Could you check a few things on this model? Use its own coordinates, in mm. Face numbers are marked on the shaded views. A direction names the side the tool comes from. Round coordinates to 2 decimals unless told otherwise and drop trailing zeros. Write each loop counter-clockwise with the first axis right and the second up, starting at its lowest first coordinate (ties: lowest second). Pieces come first, ordered by that corner, then holes. Notation, with made-up numbers: M 59.5,71 L 112.5,71 A17 cw 112.5,94 Z; hole C 42,12 d1. An arc over 180 degrees is marked long. One line per item, written item: value. Start each with the question number.
(1) I want a section at D-D on y = -66.5. Please give me the cut outline in (x, z).
(2) I want a section at A-A on z = 23. Please give me the cut outline in (x, y).
(3) I want a section at B-B on y = 32. Please give me the cut outline in (x, z).
(4) Which directions (+Z, -Z, +X, -X, +Y, -Y) give clear straight access to the entire face, cutting with the end or side of a thin tool? Please do the marked faces 1 and 2.
(5) I want a section at C-C on x = -51. Please give me the cut outline in (y, z), and give its area (3 significant figures).
(6) If I drill on L1, parallel to Y at x = 0, z = 2.4; L2, parallel to Y at x = 57, z = 4.5; L3, parallel to Y at x = 9.5, z = 23, over which ranges is the centre line in solid material (lowest first)?
(7) I'm going to push flat-ended pins straight in: pin 1 Ø12 at (x, y) = (30, 69) entering from +Z; pin 2 Ø1.5 at (x, z) = (54.5, 3.5) entering from +Y; pin 3 Ø12 at (y, z) = (12, 10) entering from +X. Where does each tip first touch, or does it pass through?
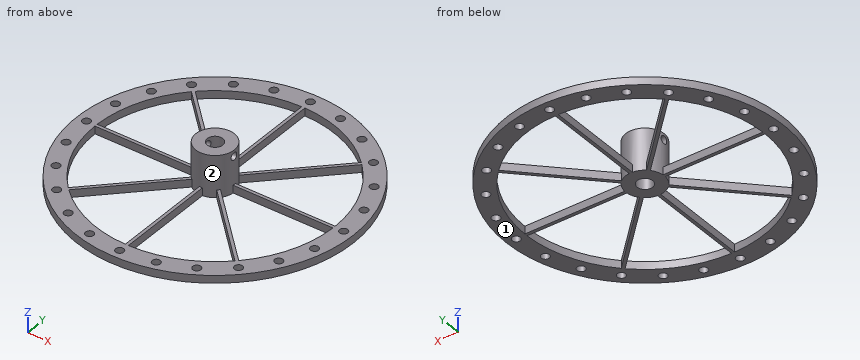
Autodesk Fusion 360 part; units mm, degrees
sketch "Sketch1" plane through (0, 0, 0) normal (0, 0, 1) x (1, 0, 0)
  line L0 (-1, 0) -> (-1, -77.5)
  line L1 (-0.4142, -1) -> (77.5, -1)
  line L2 (-1, 0) -> (-1, 77.5)
  line L3 (-0.4142, 1) -> (-55.5079, -54.0937)
  line L4 (0, 0) -> (77.5, 0) construction
  line L5 (0, 0) -> (0, 77.5) construction
  line L6 (0, 0) -> (-54.8008, -54.8008) construction
  line L7 (-2.4142, 1) -> (54.0937, -55.5079)
  line L8 (0, 0) -> (0, -77.5) construction
  line L9 (-0.4142, -1) -> (-55.5079, 54.0937)
  line L10 (0, -1) -> (-77.5, -1)
  line L11 (2.4142, 1) -> (55.5079, 54.0937)
  line L12 (0, 0) -> (77.5, 0) construction
  line L13 (0.7071, 0.7071) -> (-54.0937, 55.5079)
  line L14 (0, 0) -> (-54.8008, 54.8008) construction
  line L15 (2.4142, 1) -> (77.5, 1)
  line L16 (0, 1) -> (-77.5, 1)
  circle A0 centre (0, 0) radius 12.5
  line L17 (-2.4142, 1) -> (77.5, 1)
  line L18 (-0.4142, 1) -> (77.5, 1)
  line L19 (2.4142, -1) -> (77.5, -1)
  line L20 (-2.4142, -1) -> (77.5, -1)
  line L21 (0, 0) -> (-77.5, 0) construction
  circle A1 centre (0, 0) radius 5.05
  line L22 (1, 0) -> (1, -77.5)
  line L23 (0.4142, -1) -> (-54.0937, -55.5079)
  line L24 (0, 0) -> (54.8008, 54.8008) construction
  line L25 (1, 0) -> (1, 77.5)
  line L26 (0, 0) -> (77.5, 0) construction
  circle A2 centre (0, 0) radius 77.5
  line L27 (0, 0) -> (77.5, 0) construction
  circle A3 centre (0, 0) radius 90
  line L28 (0.4142, -1) -> (77.5, -1)
  line L29 (0, 0) -> (54.8008, -54.8008) construction
  line L30 (-2.4142, -1) -> (54.0937, 55.5079)
  line L31 (0, 0) -> (77.5, 0) construction
  line L32 (2.4142, -1) -> (55.5079, -54.0937)
  dimension "d42" = 1
  dimension "d43" = -1
  dimension "d44" = 1
  dimension "d45" = -1
  dimension "d46" = 1
  dimension "d47" = -1
  dimension "d48" = 1
  dimension "d49" = -1
  dimension "d50" = 1
  dimension "d51" = -1
  dimension "d52" = 1
  dimension "d53" = -1
  dimension "d54" = 1
  dimension "d55" = -1
  dimension "d33" = 10.1
  dimension "d35" = 180
  dimension "d37" = 155
  dimension "d38" = 45
  dimension "d39" = 45
  dimension "d40" = 135
  dimension "d41" = 135
  dimension "d56" = 25
extrude "Extrude1" add sketch "Sketch1" along normal blind 27 contours L0 A0 A1 L22 | L0 A0 A1 L23 | L3 A0 A1 L23 | L3 L10 A0 A1 | L10 L16 A0 A1 | L9 L16 A0 A1 | L9 L13 A0 A1 | L2 L13 A0 A1 | L2 A0 A1 L25 | L7 A0 A1 L22 | L7 A0 A1 L32 | A0 A1 L25 L30 | L11 A0 A1 L30 | L1 A0 L19 L20 A1 L28 L32 | L11 L15 A0 L17 L18 A1 | L1 L15 A0 L17 L18 L19 L20 A1 L28
extrude "Extrude2" add sketch "Sketch1" along normal blind 5 contours L0 A0 L22 A2 | L3 A0 L23 A2 | L10 L16 A0 A2 | L9 L13 A0 A2 | L2 A0 L25 A2 | L7 A0 A2 L32 | L11 A0 A2 L30 | L1 L15 A0 L17 L18 L19 L20 A2 L28 | A3
sketch "Sketch2" plane through (0, 0, 5) normal (0, 0, 1) x (-1, 0, 0)
  arc A0 (1, 12.4599) -> (-1, 12.4599) centre (0, 0) ccw
  line L0 (1, 12.4599) -> (1, 77.4935)
  arc A1 (54.0891, 55.5033) -> (1, 77.4935) centre (0, 0) ccw
  line L1 (54.0891, 55.5033) -> (8.1034, 9.5176)
  arc A2 (9.5176, 8.1034) -> (8.1034, 9.5176) centre (0, 0) ccw
  line L2 (9.5176, 8.1034) -> (55.5033, 54.0891)
  arc A3 (77.4935, 1) -> (55.5033, 54.0891) centre (0, 0) ccw
  line L3 (77.4935, 1) -> (12.4599, 1)
  arc A4 (12.4599, -1) -> (12.4599, 1) centre (0, 0) ccw
  line L4 (12.4599, -1) -> (77.4935, -1)
  arc A5 (55.5033, -54.0891) -> (77.4935, -1) centre (0, 0) ccw
  line L5 (55.5033, -54.0891) -> (9.5176, -8.1034)
  arc A6 (8.1034, -9.5176) -> (9.5176, -8.1034) centre (0, 0) ccw
  line L6 (8.1034, -9.5176) -> (54.0891, -55.5033)
  arc A7 (1, -77.4935) -> (54.0891, -55.5033) centre (0, 0) ccw
  line L7 (1, -77.4935) -> (1, -12.4599)
  arc A8 (-1, -12.4599) -> (1, -12.4599) centre (0, 0) ccw
  line L8 (-1, -12.4599) -> (-1, -77.4935)
  arc A9 (-54.0891, -55.5033) -> (-1, -77.4935) centre (0, 0) ccw
  line L9 (-54.0891, -55.5033) -> (-8.1034, -9.5176)
  arc A10 (-9.5176, -8.1034) -> (-8.1034, -9.5176) centre (0, 0) ccw
  line L10 (-9.5176, -8.1034) -> (-55.5033, -54.0891)
  arc A11 (-77.4935, -1) -> (-55.5033, -54.0891) centre (0, 0) ccw
  line L11 (-77.4935, -1) -> (-12.4599, -1)
  arc A12 (-12.4599, 1) -> (-12.4599, -1) centre (0, 0) ccw
  line L12 (-12.4599, 1) -> (-77.4935, 1)
  arc A13 (-55.5033, 54.0891) -> (-77.4935, 1) centre (0, 0) ccw
  line L13 (-55.5033, 54.0891) -> (-9.5176, 8.1034)
  arc A14 (-8.1034, 9.5176) -> (-9.5176, 8.1034) centre (0, 0) ccw
  line L14 (-8.1034, 9.5176) -> (-54.0891, 55.5033)
  arc A15 (-1, 77.4935) -> (-54.0891, 55.5033) centre (0, 0) ccw
  line L15 (-1, 77.4935) -> (-1, 12.4599)
  circle A16 centre (0, 0) radius 90
  line L16 (-77.5, 0) -> (-83.75, 0) construction
  circle A17 centre (-83.75, 0) radius 2.65
  point P0 (-77.5, 0)
  dimension "d28" = 6.25
  dimension "d29" = 5.3
hole "Hole1" at (83.75, 0, 5) direction (0, 0, -1) diameter 5.3 depth 10 tip angle 180
pattern_circular "C-Pattern1" count 24 over 360 about axis through (0, 0, 0) along (0, 0, 1) of "Hole1"
ref_plane "WorkPlane1" through (12.5, 0, 19.1773) normal (1, 0, 0) x (0, -1, 0)
ref_plane "WorkPlane2" through (-12.5, 0, 14.5915) normal (-1, 0, 0) x (0, 1, 0)
ref_plane "WorkPlane3" through (0, 0, 14.5915) normal (-1, 0, 0) x (0, 1, 0)
sketch "Sketch3" plane through (0, 0, 14.5915) normal (-1, 0, 0) x (0, 1, 0)
  line L0 (-12.5, -12.4085) -> (12.5, -12.4085)
  line L1 (0, -12.4085) -> (0, -8.4085)
  circle A0 centre (0, -8.4085) radius 2.5
  dimension "d59" = 4
  dimension "d60" = 5
extrude "Extrude3" cut sketch "Sketch3" along normal blind 16 and the other way blind 18
equation "d28 = ( 12.500 / 2 ) * 1 mm"
Found:
1. outline: M -60.64,0 L -39.8,0 L -39.8,5 L -60.64,5 Z; M -1,0 L 1,0 L 1,5 L -1,5 Z; M 39.8,0 L 60.64,0 L 60.64,5 L 39.8,5 Z
2. outline: M -12.25,-2.5 A12.5 ccw 12.25,-2.5 L 4.39,-2.5 A5.05 cw -4.39,-2.5 Z; M -12.25,2.5 L -4.39,2.5 A5.05 cw 4.39,2.5 L 12.25,2.5 A12.5 ccw Z
3. outline: M -84.12,0 L -70.59,0 L -70.59,5 L -84.12,5 Z; M -33.41,0 L -30.59,0 L -30.59,5 L -33.41,5 Z; M -1,0 L 1,0 L 1,5 L -1,5 Z; M 30.59,0 L 33.41,0 L 33.41,5 L 30.59,5 Z; M 70.59,0 L 84.12,0 L 84.12,5 L 70.59,5 Z
4. face 1: -Z, +X, -X, +Y, -Y
4. face 2: +Z
5. outline: M -74.16,0 L -58.35,0 L -58.35,5 L -74.16,5 Z; M -52.41,0 L -49.59,0 L -49.59,5 L -52.41,5 Z; M -1,0 L 1,0 L 1,5 L -1,5 Z; M 49.59,0 L 52.41,0 L 52.41,5 L 49.59,5 Z; M 58.35,0 L 74.16,0 L 74.16,5 L 58.35,5 Z
5. area: 196 mm²
6. L1: y = -90 to -86.4, -81.1 to -5.05, 5.05 to 81.1, 86.4 to 90
6. L2: y = -69.65 to -60.67, -57.77 to -52.51, -1 to 1, 52.51 to 57.77, 60.67 to 69.65
6. L3: y = -8.12 to -2.5, 2.5 to 8.12
7. pin 1: stops at z = 5
7. pin 2: stops at y = 72.19
7. pin 3: stops at x = 89.58
